Input: dimensioned drawing with shaded views. Units: mm. Origin: part minimum x, y, z. A direction names the side the tool comes from. Round coordinates to 2 decimals unless told otherwise and drop trailing zeros. Loops run counter-clockwise (first coordinate to the right, second up) from the corner with the lowest first, then second, coordinate; pieces in that order, holes last. Notation, with made-up numbers: (-20.75, 77.25) -> (6.25, 77.25) arc R34 ccw to (6.25, 108.25) -> close; hole circle Ø10 at (-25.5, 51.5). An arc over 180 degrees is marked (long way). Answer as a JSON object with one key per item and string values.
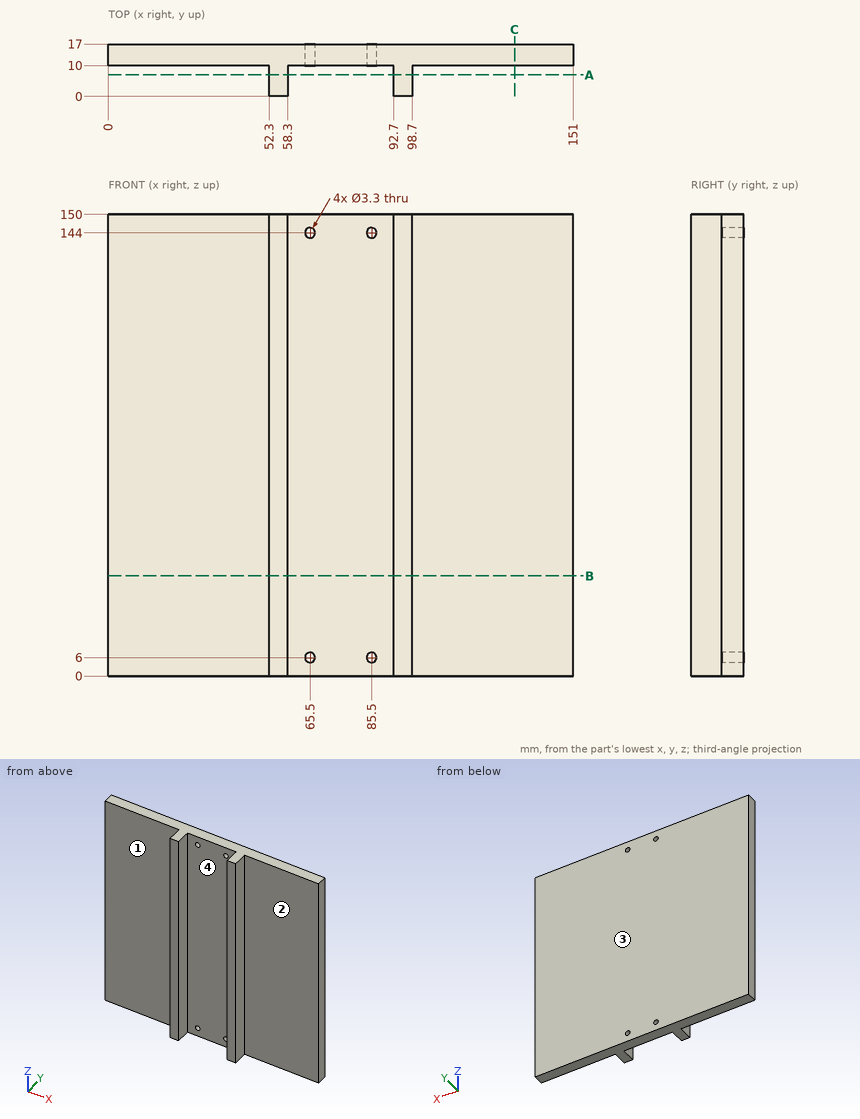
1) Section B-B, the plane z = 32.5. Output: boundary loops of the cut face in (x, y).
Output:
{"outline": "(0, 10) -> (52.3, 10) -> (52.3, 0) -> (58.3, 0) -> (58.3, 10) -> (92.7, 10) -> (92.7, 0) -> (98.7, 0) -> (98.7, 10) -> (151, 10) -> (151, 17) -> (0, 17) -> close"}
2) Ray query, probe 1 along Z at (x, y) = (65.5, 14); probe 2 along X at (y, z) = (12.25, 144); probe 3 along X at (y, z) = (6, 141.5). Return the intervals inside material, ascending.
Output:
{"probe 1": "z = 0 to 4.35, 7.65 to 142.35, 145.65 to 150", "probe 2": "x = 0 to 63.85, 67.15 to 83.85, 87.15 to 151", "probe 3": "x = 52.3 to 58.3, 92.7 to 98.7"}
3) Section A-A, the plane y = 7. Output: boundary loops of the cut face in (x, z), plus the area to 3 significant figures.
Output:
{"outline": "(52.3, 0) -> (58.3, 0) -> (58.3, 150) -> (52.3, 150) -> close; (92.7, 0) -> (98.7, 0) -> (98.7, 150) -> (92.7, 150) -> close", "area": "1,800 mm^2"}
4) Contact query for flat-ended pins moving along their axis: P1, Ø10, axis at x = 54.5, y = 8, coming from the -Z side; P2, Ø1, axis at y = 6.5, z = 40, coming from the +X side; P3, Ø8, axis at y = 2.5, z = 101.5, coming from the -X side; P4, Ø15.5, axis at x = 13.5, z = 75.5, coming from the -Y side. Output: stop coordinate, or through.
Output:
{"P1": "stops at z = 0", "P2": "stops at x = 98.7", "P3": "stops at x = 52.3", "P4": "stops at y = 10"}
5) Section C-C, the plane x = 132. Output: boundary loops of the cut face in (y, z), plus the area to 3 significant figures.
Output:
{"outline": "(10, 0) -> (17, 0) -> (17, 150) -> (10, 150) -> close", "area": "1,050 mm^2"}
6) Draft query along X for the marked faces 3 and 4. Return one class per face: +X half, -X half, draft (parallel to the pull), parting line (faces both ways), or undercut.
Output:
{"face 3": "draft", "face 4": "undercut"}
7) Reachability of the marked faces 1 and 2 from +Z, -Z, +X, -X, +Y, -Y: full face, straight path, thin tool, end or side. Return the list, or none.
Output:
{"face 1": "+Z, -Z, -X, -Y", "face 2": "+Z, -Z, +X, -Y"}
